Input: dimensioned drawing with shaded views. Units: mm. Origin: part minimum x, y, z. A direction names the side the tool comes from. Round coordinates to 2 decimals unless told otherwise and drop trailing zeros. Order: outer loops, then holes, each group sorted by start corner. A loop starts at its lowest first (then second) coordinate and runs counter-clockwise, first axis right, second up. Notation, with made-up numbers: M 87,12 L 121,12 A25 cw 121,41 Z; hole C 70,-1 d11. An arc over 180 degrees is marked long. Answer as CSV lines item,"result". Start each with the question number.
Item 1: Line query: line 1 (X direction, y = 7, z = 5.5); line 2 (Z direction, x = 7, y = 4.75); line 3 (Y direction, x = 3, z = 11.25). Output: solid intervals per line, ascending. Write a range as [from, to].
Item 2: Pull-direction query (X, two-part tool) for the marked faces 1, 2 and 3; classes: +X half, -X half, draft (parallel to the pull), parting line (faces both ways), or undercut.
Item 3: Section query A-A on x = 7. Return the cut outline in (y, z).
Item 4: Section query B-B on y = 8.5. Return the cut outline in (x, z), plus the area to 3 significant figures.
Item 5: Set-up query: the marked faces 4 and 5. Return all of +Z, -Z, +X, -X, +Y, -Y with unobstructed straight access to the full face (end or side cutting, diameter ignored); none if empty.
Item 6: Section query C-C on y = 5.75. Return the cut outline in (x, z).
Item 7: First-contact query: P1, Ø1, axis at y = 4, z = 10, coming from the +X side; P2, Ø3, axis at x = 9.5, y = 7, coming from the +Z side; P3, Ø4, axis at x = 6.5, z = 4, coming from the +Y side. Flat tips, straight axial feed; report the tip coordinate or a pass-through.
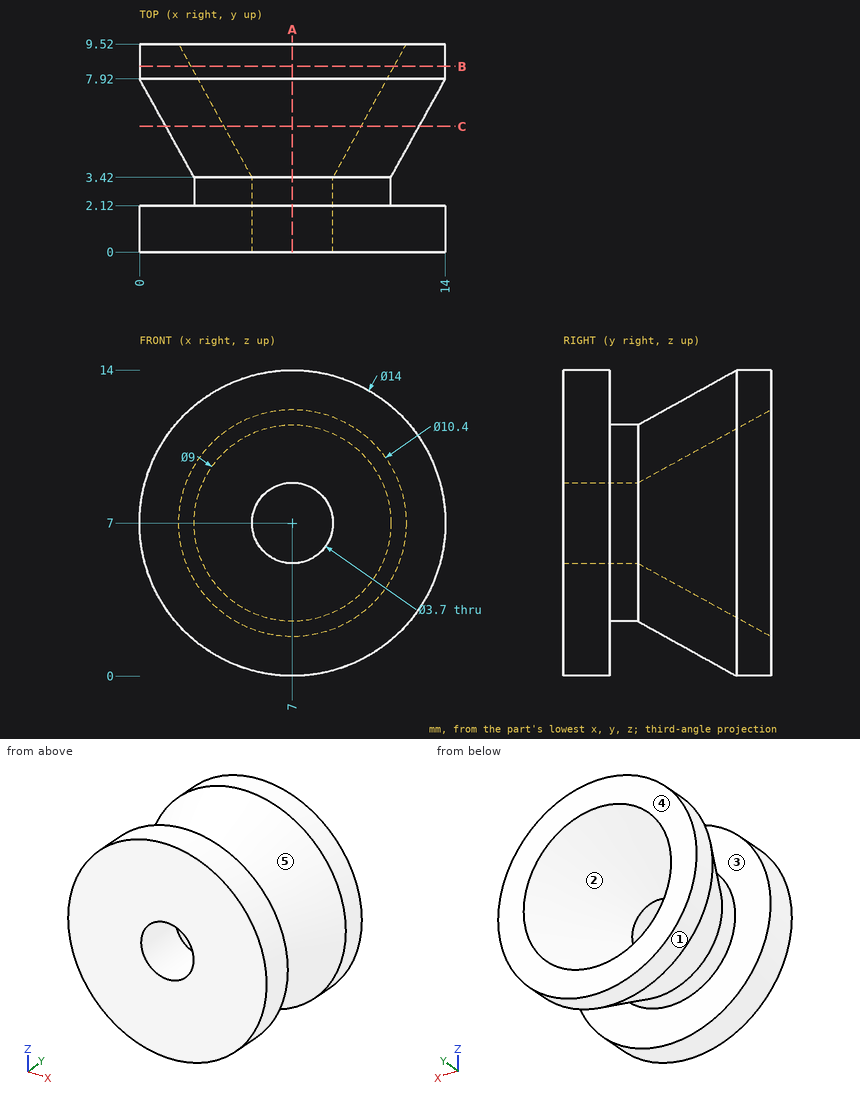
Results:
1,line 1,"[0.69, 3.49], [10.51, 13.31]"
1,line 2,"[1.76, 4.42], [9.58, 12.24]"
1,line 3,"[0, 2.12], [5.83, 9.52]"
2,face 1,"parting line"
2,face 2,"undercut"
2,face 3,"draft"
3,outline,"M 0,0 L 2.12,0 L 2.12,2.5 L 3.42,2.5 L 7.92,0 L 9.52,0 L 9.52,1.8 L 3.42,5.15 L 0,5.15 Z; M 0,8.85 L 3.42,8.85 L 9.52,12.2 L 9.52,14 L 7.92,14 L 3.42,11.5 L 2.12,11.5 L 2.12,14 L 0,14 Z"
4,outline,"C 7,7 d14; hole C 7,7 d9.28"
4,area,"86.3 mm^2"
5,face 4,"+Z, -Z, +X, -X, +Y"
5,face 5,"none"
6,outline,"C 7,7 d11.59; hole C 7,7 d6.26"
7,P1,"x = 11.26"
7,P2,"z = 13.88"
7,P3,"y = 9.23"
